The listing builds one solid part. Answer for the finished solid, in the listing's coordinates (mm). A direction names the side the tool comes from. Round coordinates to 2 decimals unless told otherwise and drop trailing zeros. Order: outer loops, then holes, each group sorted by start corner. A loop starts at its lowest first (then second) coordinate and runs counter-clockwise, first axis right, second up. Notation, with made-up numbers: M -33.5,42.5 L -0.5,42.5 A18 ccw -0.5,60.5 Z; hole C 89.5,58.5 d7. An arc over 180 degrees is marked long. Write item = value, one per line. Start each with the question number.
(1) A cutting plane is placed at B-B, the plane z = 3.45. Determine the outline of the cut face in (x, y) (3 decimals).
(2) For a pull along Y with two mould halves and no side action, classify faces 1 (the face through (22, 25, 0)), 2 (the face through (14.59, 44.31, 2.46)), 3 (the face through (23.505, 50.202, 0.986)) as released by +Y, released by -Y, zero draft, split by the parting line, or undercut.
(3) A cutting plane is placed at C-C, the plane x = 11. Determine the outline of the cut face in (y, z), and give its area (3 significant figures).
(4) A cutting plane is placed at A-A, the plane y = 15. Determine the outline of the cut face in (x, z).
(5) A cutting plane is placed at D-D, the plane y = 45.5. Determine the outline of the cut face in (x, z).
(6) Straight lines are drawn through the part: probe 1 along Y at (x, z) = (37, 1.7); probe 2 along X at (y, z) = (42, 2.15); probe 3 along X at (y, z) = (19, 1). For each, find the intervals that lie inside material, in ascending order. Write a range as from..to.
(7) Which of the six approach directions +Z, -Z, +X, -X, +Y, -Y give full straight-line access (tool end or side, diameter ignored) to faces 4 (the face through (23.41, 39.1, 3.52)), 5 (the face through (24.931, 39, 1)), 6 (the face through (6.434, 50.28, 0.986))?
(8) Each of these flat-tipped pins is pushed along its axis until it touches: pin 1 (1.6 mm diameter, centred on y = 41, z = 1.5, fed in from +X); pin 2 (0.6 mm diameter, centred on x = 35, z = 1, fed in from +Y). Where does it stop, or does it pass through?
from build123d import *

# Parameters (mm, degrees)
F0_R     = 2.625
F1_DEPTH = 5
F2_SIZE  = 3


with BuildPart() as f1:
    # F0 (on Top) → F1 (new body)
    with BuildSketch(Plane.XY):
        with BuildLine():
            ThreePointArc((4.930798, 11.705586), (6.395264, 8.170052), (9.930798, 6.705586))
            Line((9.930798, 6.705586), (44.930798, 6.705586))
            ThreePointArc((44.930798, 6.705586), (48.466332, 8.170052), (49.930798, 11.705586))
            Line((49.930798, 11.705586), (49.930798, 21.705586))
            ThreePointArc((49.930798, 21.705586), (48.466332, 25.241119), (44.930798, 26.705586))
            Line((44.930798, 26.705586), (29.930798, 26.705586))
            ThreePointArc((29.930798, 26.705586), (26.395264, 28.170052), (24.930798, 31.705586))
            Line((24.930798, 31.705586), (24.930798, 46.705586))
            ThreePointArc((24.930798, 46.705586), (23.466332, 50.241119), (19.930798, 51.705586))
            Line((19.930798, 51.705586), (9.930798, 51.705586))
            ThreePointArc((9.930798, 51.705586), (6.395264, 50.241119), (4.930798, 46.705586))
            Line((4.930798, 46.705586), (4.930798, 26.705586))
            Line((4.930798, 26.705586), (4.930798, 11.705586))
        make_face()
        with Locations((14.930798, 16.705586)):
            Circle(F0_R, mode=Mode.SUBTRACT)
        with Locations((39.930798, 16.705586)):
            Circle(F0_R, mode=Mode.SUBTRACT)
        with Locations((14.930798, 41.705586)):
            Circle(F0_R, mode=Mode.SUBTRACT)
    extrude(amount=F1_DEPTH)

    # F2
    f2_edges = [f1.edges().sort_by_distance(p)[0] for p in [
        (14.930798, 51.705586, 5),
        (23.466332, 50.241119, 5),
        (24.930798, 39.205586, 5),
        (26.395264, 28.170052, 5),
        (37.430798, 26.705586, 5),
        (48.466332, 25.241119, 5),
        (49.930798, 16.705586, 5),
        (48.466332, 8.170052, 5),
        (27.430798, 6.705586, 5),
        (6.395264, 8.170052, 5),
        (4.930798, 29.205586, 5),
        (6.395264, 50.241119, 5),
    ]]
    chamfer(f2_edges, length=F2_SIZE)


solid = f1.part
Reported:
q1.outline = M 6.381,11.706 A3.55 ccw 9.931,8.156 L 44.931,8.156 A3.55 ccw 48.481,11.706 L 48.481,21.706 A3.55 ccw 44.931,25.256 L 29.931,25.256 A6.45 cw 23.481,31.706 L 23.481,46.706 A3.55 ccw 19.931,50.256 L 9.931,50.256 A3.55 ccw 6.381,46.706 Z; hole C 14.931,16.706 d5.25; hole C 14.931,41.706 d5.25; hole C 39.931,16.706 d5.25
q2.face_1 = zero draft
q2.face_2 = undercut
q2.face_3 = released by +Y
q3.outline = M 6.71,0 L 51.71,0 L 51.71,2 L 48.71,5 L 9.71,5 L 6.71,2 Z
q3.area = 216 mm²
q4.outline = M 4.93,0 L 12.94,0 L 12.94,5 L 7.93,5 L 4.93,2 Z; M 16.93,0 L 37.94,0 L 37.94,5 L 16.93,5 Z; M 41.93,0 L 49.93,0 L 49.93,2 L 46.93,5 L 41.93,5 Z
q5.outline = M 4.93,0 L 24.93,0 L 24.93,2 L 21.93,5 L 7.93,5 L 4.93,2 Z
q6.probe_1 = 6.71..26.71
q6.probe_2 = 5.08..12.32, 17.54..24.78
q6.probe_3 = 4.93..13.66, 16.21..38.66, 41.21..49.93
q7.face_4 = +Z, +X, +Y
q7.face_5 = +Z, -Z, +X, +Y
q7.face_6 = +Z, -Z, -X, +Y
q8.pin_1 = 24.93
q8.pin_2 = 26.71
